Source: CAD feature listing. Evaluate the final solid. Frame: model axes, mm. A direction names the side the tool comes from. Round coordinates to 2 decimals unless told otherwise and drop trailing zeros. Order: outer loops, then holes, each group sorted by start corner. A loop starts at its lowest first (then second) coordinate and runs counter-clockwise, first axis right, second up. Notation, with made-up numbers: (68, -39) - (110, -39) arc R33 ccw to (110, -9) - close; hole circle Ø3 at (-14.5, -22). An arc over 180 degrees is marked (long way). Return JSON: item names as keys, results as strings. Group by question number.
1) Ray query, line 1 (Y direction, x = 0.5, z = -4.75); line 2 (X direction, y = 8, z = 2); line 3 (X direction, y = -10, z = -0.75). Return the intervals inside material, ascending. Write a range as from..to.
2) Access query for faces 4 (the flat face through (0, 8, -4.076)), 5 (the flat face through (-2, 17, -2)), 6 (the flat face through (2, 7, -0.126)). Directions: +Z, -Z, +X, -X, +Y, -Y. A direction counts if a zero-diameter tool reaches every point of the face in a straight line with its end or side. Return the directions, or none.
3) Section C-C, the plane z = -3.75. Return loops of the section in (x, y), plus the area to 3 significant figures.
4) Contact query for flat-ended pins moving along their axis: P1, Ø0.8, axis at x = -0.5, z = -1.5, coming from the -Y side; P2, Ø1, axis at x = 4.5, z = -3, coming from the +Y side; P3, Ø5.5, axis at x = -0.5, y = 4.5, coming from the -Z side. Output: stop coordinate, or through.
5) Section B-B, the plane x = -2.75. Return loops of the section in (y, z).
6) Mould query, pull axis Y, two halves, no side actions, for faces 1 (the cylindrical face through (0.57, 0.59, -1.96)), 2 (the flat face through (-3, 7, -1.126)), 3 (the flat face through (2.5, -2, -0.5)). Classes: pulls with the +Y half, pulls with the -Y half, needs draft (parallel to the pull), parting line crosses it, or undercut.
7) Section A-A, the plane y = 13. Return loops of the section in (x, z).
8) Section D-D, the plane x = 2.75. Return loops of the section in (y, z), plus the area to 3 significant figures.
```python
from build123d import *

# Parameters (mm, degrees)
SKETCH_2_W          = 6.9
SKETCH_2_H          = 6.9
EXTRUDE_1_DEPTH     = 17
SKETCH_3_R          = 2
EXTRUDE_2_DEPTH     = 5
SKETCH_4_W          = 1
SKETCH_4_H          = 13.542540749
CUT_EXTRUDE_1_DEPTH = 15
SKETCH_5_R          = 6
EXTRUDE_3_DEPTH     = 2
SKETCH_6_R          = 2.25
EXTRUDE_4_DEPTH     = 10
SKETCH_7_R          = 1.5
CUT_EXTRUDE_2_DEPTH = 25.542541


with BuildPart() as part:
    # 草图2 → 凸台-拉伸1 (new body)
    with BuildSketch(Plane(origin=(0, 0, 0), x_dir=(1, 0, 0), z_dir=(0, 1, 0))):
        with Locations((-0.118382353, 0.625735294)):
            Rectangle(SKETCH_2_W, SKETCH_2_H)
    extrude(amount=EXTRUDE_1_DEPTH)

    # 草图3 → 凸台-拉伸2 (add)
    with BuildSketch(Plane(origin=(0, 17, 0), x_dir=(1, 0, 0), z_dir=(0, 1, 0))):
        with Locations((-0.118382353, 0.625735294)):
            Circle(SKETCH_3_R)
    extrude(amount=EXTRUDE_2_DEPTH)

    # 草图4 → 切除-拉伸1 (cut)
    with BuildSketch(Plane.ZY.offset(3.568382353)):
        with Locations((-0.625735294, 6.771270375)):
            Rectangle(SKETCH_4_W, SKETCH_4_H)
    extrude(amount=-CUT_EXTRUDE_1_DEPTH, mode=Mode.SUBTRACT)

    # 草图5 → 凸台-拉伸3 (add)
    with BuildSketch(Plane.XZ):
        with Locations((-0.118382353, -0.625735294)):
            Circle(SKETCH_5_R)
    extrude(amount=EXTRUDE_3_DEPTH)

    # 草图6 → 凸台-拉伸4 (add)
    with BuildSketch(Plane.XZ.offset(2)):
        with Locations((-0.118382353, -0.625735294)):
            Circle(SKETCH_6_R)
    extrude(amount=EXTRUDE_4_DEPTH)

    # 草图7 → 切除-拉伸2 (cut)
    with BuildSketch(Plane.XZ.offset(12)):
        with Locations((-0.118382353, -0.625735294)):
            Circle(SKETCH_7_R)
    extrude(amount=-CUT_EXTRUDE_2_DEPTH, mode=Mode.SUBTRACT)


solid = part.part
```
Geometry check:
{
 "1": {"line 1": "-2..0", "line 2": "-3.57..3.33", "line 3": "-2.36..-1.61, 1.38..2.13"},
 "2": {"face 4": "-Z, +X, -X, +Y", "face 5": "+Y", "face 6": "+X, -X"},
 "3": {"outline": "(-5.24, -2) - (5, -2) - (5, 0) - (3.33, 0) - (3.33, 17) - (-3.57, 17) - (-3.57, 0) - (-5.24, 0) - close", "area": "138 mm2"},
 "4": {"P1": "y = 13.54", "P2": "y = 0", "P3": "z = -4.08"},
 "5": {"outline": "(-2, -6.02) - (0, -6.02) - (0, -4.08) - (17, -4.08) - (17, 2.82) - (0, 2.82) - (0, 4.77) - (-2, 4.77) - close; hole (0, -1.13) - (13.54, -1.13) - (13.54, -0.13) - (0, -0.13) - close"},
 "6": {"face 1": "needs draft", "face 2": "undercut", "face 3": "pulls with the -Y half"},
 "7": {"outline": "(-3.57, -4.08) - (3.33, -4.08) - (3.33, -1.13) - (1.3, -1.13) arc R1.5 cw to (-1.53, -1.13) - (-3.57, -1.13) - close; (-3.57, -0.13) - (-1.53, -0.13) arc R1.5 cw to (1.3, -0.13) - (3.33, -0.13) - (3.33, 2.82) - (-3.57, 2.82) - close"},
 "8": {"outline": "(-2, -5.9) - (0, -5.9) - (0, -4.08) - (17, -4.08) - (17, 2.82) - (0, 2.82) - (0, 4.64) - (-2, 4.64) - close; hole (0, -1.13) - (13.54, -1.13) - (13.54, -0.13) - (0, -0.13) - close", "area": "125 mm2"}
}
